CAD build for the part. Positions are in the model's coordinates, mm. Face numbers are marked on the shaded views. A direction names the side the tool comes from. Coordinates: 2 decimals unless noted, no trailing zeros. Order: outer loops, then holes, each group sorted by start corner. A loop starts at its lowest first (then second) coordinate and runs counter-clockwise, first axis right, second up. Notation, with made-up numbers: M 22.5,65.25 L 42.5,65.25 A24 cw 42.5,95.25 Z; hole C 5.5,-19.5 d4. An arc over 180 degrees is marked long. Write item = value, one per line.
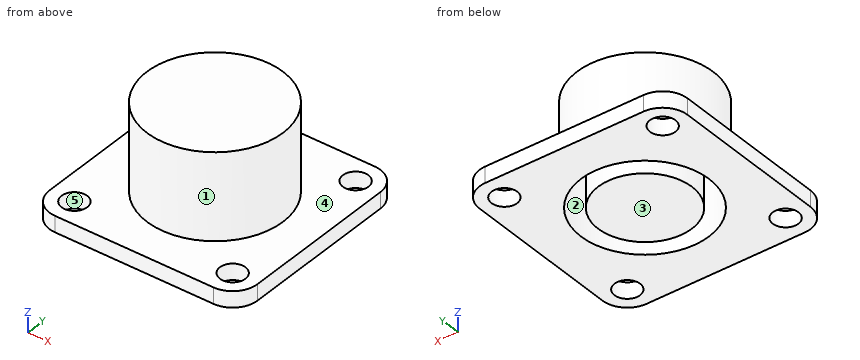
from build123d import *

# Parameters (mm, degrees)
SKETCH1_W                = 26
SKETCH1_H                = 26
BOSS_EXTRUDE1_DEPTH      = 2
FILLET1_R                = 3.1
SKETCH3_R                = 8.5
BOSS_EXTRUDE2_DEPTH      = 12.8
M3_CLEARANCE_HOLE1_D     = 3.2
M3_CLEARANCE_HOLE1_DEPTH = 5
M3_CLEARANCE_HOLE1_TIP   = 0.96137699
SKETCH7_R                = 8
SKETCH7_R_2              = 5.85
CUT_EXTRUDE1_DEPTH       = 11.8


with BuildPart() as part:
    # Sketch1 → Boss-Extrude1 (new body)
    with BuildSketch(Plane.XY):
        Rectangle(SKETCH1_W, SKETCH1_H)
    extrude(amount=BOSS_EXTRUDE1_DEPTH)

    # Fillet1
    fillet1_edges = [part.edges().sort_by_distance(p)[0] for p in [
        (13, -13, 1),
        (-13, -13, 1),
        (-13, 13, 1),
        (13, 13, 1),
    ]]
    fillet(fillet1_edges, radius=FILLET1_R)

    # Sketch3 → Boss-Extrude2 (add)
    with BuildSketch(Plane.XY):
        Circle(SKETCH3_R)
    extrude(amount=BOSS_EXTRUDE2_DEPTH)

    # M3 Clearance Hole1
    with Locations(Plane(origin=(0, 0, 0), x_dir=(-1, 0, 0), z_dir=(0, 0, -1))):
        with Locations((9.9, 9.9), (9.9, -9.9), (-9.9, -9.9), (-9.9, 9.9)):
            Hole(M3_CLEARANCE_HOLE1_D / 2, depth=M3_CLEARANCE_HOLE1_DEPTH)
            with Locations((0, 0, -(M3_CLEARANCE_HOLE1_DEPTH + M3_CLEARANCE_HOLE1_TIP / 2))):  # 118° drill point
                Cone(0, M3_CLEARANCE_HOLE1_D / 2, M3_CLEARANCE_HOLE1_TIP, mode=Mode.SUBTRACT)

    # Sketch7 → Cut-Extrude1 (cut)
    with BuildSketch(Plane(origin=(0, 0, 0), x_dir=(-1, 0, 0), z_dir=(0, 0, -1))):
        Circle(SKETCH7_R)
        Circle(SKETCH7_R_2, mode=Mode.SUBTRACT)
    extrude(amount=-CUT_EXTRUDE1_DEPTH, mode=Mode.SUBTRACT)


solid = part.part
(1) Slice it at C-C, the plane z = 9.5. Write the cut outline in (x, y).
Evaluation:
outline = C 0,0 d17; C 0,0 d11.7; hole C 0,0 d16
(2) Slice it at B-B, the plane y = 10.5. Write the cut outline in (x, z), then the cut area to 3 significant figures.
Evaluation:
outline = M -12.94,0 L -11.38,0 L -11.38,2 L -12.94,2 Z; M -8.42,0 L 8.42,0 L 8.42,2 L -8.42,2 Z; M 11.38,0 L 12.94,0 L 12.94,2 L 11.38,2 Z
area = 39.9 mm²
(3) Pull direction Y, two halves, no side cores. Call the marked faces 1, 2 and 3: +Y half, -Y half, draft (parallel to the pull), parting line (faces both ways), or undercut.
Evaluation:
face_1 = parting line
face_2 = undercut
face_3 = draft
(4) Tool access for the marked faces 4 and 5: list every direction of +Z, -Z, +X, -X, +Y, -Y with a clear straight run to the whole face (end or side of a thin tool).
Evaluation:
face_4 = +Z
face_5 = +Z, -Z
(5) Wall check: line 1 (Y direction, x = -9.9, z = 0.8); line 2 (Y direction, x = 0, z = 3.5); line 3 (X direction, y = -1.75, z = 5.5). Give the ranges that are in metal, low to high. Write a range as from..to.
Evaluation:
line_1 = -13..-11.5, -8.3..8.3, 11.5..13
line_2 = -8.5..-8, -5.85..5.85, 8..8.5
line_3 = -8.32..-7.81, -5.58..5.58, 7.81..8.32
(6) Slice it at A-A, the plane z = 1.25. Write the cut outline in (x, y), then the cut area to 3 significant figures.
Evaluation:
outline = M -13,-9.9 A3.1 ccw -9.9,-13 L 9.9,-13 A3.1 ccw 13,-9.9 L 13,9.9 A3.1 ccw 9.9,13 L -9.9,13 A3.1 ccw -13,9.9 Z; C 0,0 d11.7; hole C -9.9,-9.9 d3.2; hole C -9.9,9.9 d3.2; hole C 0,0 d16; hole C 9.9,-9.9 d3.2; hole C 9.9,9.9 d3.2
area = 542 mm²
(7) Pin check, flat tips, straight feed: pin 1 Ø3 at (x, y) = (9.9, 9.9) entering from +Z; pin 2 Ø1 at (y, z) = (3.5, 7) entering from -X; pin 3 Ø5 at (x, z) = (10, 9) entering from +Y; pin 4 Ø4 at (x, y) = (7, -8.5) entering from +Z. Stop position of each tip, or through.
Evaluation:
pin_1 = through
pin_2 = -7.95
pin_3 = 4
pin_4 = 2
(8) Slice it at D-D, the plane x = 0. Write the cut outline in (y, z).
Evaluation:
outline = M -13,0 L -8,0 L -8,11.8 L -5.85,11.8 L -5.85,0 L 5.85,0 L 5.85,11.8 L 8,11.8 L 8,0 L 13,0 L 13,2 L 8.5,2 L 8.5,12.8 L -8.5,12.8 L -8.5,2 L -13,2 Z
